Model file for the job. Use its own axes, mm. A direction names the side the tool comes from. Give positions to 0.01 mm unless a question says otherwise; leave off trailing zeros. Write each loop counter-clockwise with the first axis right and the second up, starting at its lowest first coordinate (ties: lowest second). Pieces come first, ordered by that corner, then holes. Notation, with made-up numbers: (32, 50) - (55, 50) arc R8 cw to (55, 63) - close; hole circle Ø5 at (59.5, 44). An arc over 180 degrees is marked (long way). One line per item, written item: value. Start each with the question number.
(1) Probe L1, parallel to X at y = 0.25, z = 0.1; L2, parallel to Y at x = -0.9, z = 1.55; L3, parallel to Y at x = -1.15, z = -0.1. List the from-to ranges inside material, lowest first.
(2) Mould opens along X. For faces 1 (the face through (0.32, -7.89, -1.43)), 2 (the face through (-1.2, 0, -1.2)), 3 (the face through (0, 2, -1.225)) say: pulls with the +X half, pulls with the -X half, needs draft (parallel to the pull), parting line crosses it, or undercut.
(3) Cut at C-C, the plane y = -14.75. List the corners of the cut face in (x, z) (3 decimals).
(4) Drop flat-ended pins along their axis: P1, Ø1, axis at y = -1.5, z = -1.5, coming from the -X side; P2, Ø2, axis at x = 2, y = -5.5, coming from the +Z side. Give the stop position or say it passes through.
(5) Cut at B-B, the plane x = 0. List the corners of the cut face in (y, z) (3 decimals), and give its area (3 significant figures).
(6) 3-axis set-ups, long thin cutter, end or side, ignore diameter. For faces 4 (the face through (-1.07, 2.01, -0.6)), 5 (the face through (0, 3, -1.5)): which of +Z, -Z, +X, -X, +Y, -Y reach the whole face in a straight line?
Autodesk Inventor part; units mm, degrees
ref_plane "YZ Plane" through (0, 0, 0) normal (1, 0, 0) x (0, 1, 0)
ref_plane "XZ Plane" through (0, 0, 0) normal (0, 1, 0) x (-1, 0, 0)
ref_plane "XY Plane" through (0, 0, 0) normal (0, 0, 1) x (1, 0, 0)
sketch "Sketch1" plane through (0, 0, 0) normal (0, 1, 0) x (-1, 0, 0)
  circle A0 centre (0, 0) radius 1.465
  circle A1 centre (0, 0) radius 2.75
  line L0 (0.7073, -1.225) -> (-0.7073, -1.225)
  line L1 (-0.7073, -1.225) -> (-1.4145, 0)
  line L2 (-1.4145, 0) -> (-0.7073, 1.225)
  line L3 (-0.7073, 1.225) -> (0.7073, 1.225)
  line L4 (0.7073, 1.225) -> (1.4145, 0)
  line L5 (1.4145, 0) -> (0.7073, -1.225)
  dimension "d0" = 2.93
  dimension "d1" = 5.5
  dimension "d8" = 2.45
extrude "Extrusion1" add sketch "Sketch1" along normal blind 3 contours A0 | A1 | L0 L1 L2 L3 L4 L5
extrude "Extrusion2" add sketch "Sketch1" against normal blind 16 contours A0 | L0 L1 L2 L3 L4 L5
extrude "Extrusion3" cut sketch "Sketch1" against normal blind 2 from surface at 3 contours L0 L1 L2 L3 L4 L5
fillet "Fillet1" radius 0.5 1 edges at (2.75, 3, 0)
thread "Thread2"
equation "\"d4\" = length"
equation "\"length\" = 16"
properties part number "M3x16"
Answers follow:
1. L1: x = -2.75 to 2.75
1. L2: y = 0 to 3
1. L3: y = -16 to 1
2. face 1: parting line crosses it
2. face 2: needs draft
2. face 3: undercut
3. outline: circle Ø2.93 at (0, 0)
4. P1: stops at x = -1.07
4. P2: stops at z = 1.07
5. outline: (-16, -1.465) - (0, -1.465) - (0, -2.75) - (2.5, -2.75) arc R0.5 ccw to (3, -2.25) - (3, -1.225) - (1, -1.225) - (1, 1.225) - (3, 1.225) - (3, 2.25) arc R0.5 ccw to (2.5, 2.75) - (0, 2.75) - (0, 1.465) - (-16, 1.465) - close
5. area: 58.4 mm²
6. face 4: +Y
6. face 5: +Z, -Z, +X, -X, +Y
